Work out the finished part from the listing and answer in its coordinate system (mm). Face numbers are marked on the shaded views. A direction names the side the tool comes from. Give positions to 0.01 mm unless a question says otherwise; leave off trailing zeros. Order: outer loops, then holes, each group sorted by start corner. A loop starts at its lowest first (then second) coordinate and runs counter-clockwise, first axis right, second up. Notation, with made-up numbers: (-35, 24.5) -> (-15, 24.5) arc R21 cw to (-15, 38.5) -> close; hole circle Ø9 at (-28.75, 32.25). An arc over 180 degrees is marked (long way). Use a Markdown table: item, result. Add a question column.
```python
from build123d import *

# Parameters (mm, degrees)
CROQUIS3_W            = 395
CROQUIS3_H            = 35
REVOLUCI_N1_ANGLE     = 90
CROQUIS5_W            = 35
CROQUIS5_H            = 35
REVOLUCI_N3_ANGLE     = 90
CORTAR_EXTRUIR5_DEPTH = 360


with BuildPart() as part:
    # Croquis3 → Revolución1 (revolve)
    with BuildSketch(Plane(origin=(0, 0, 0), x_dir=(0, 0, -1), z_dir=(1, 0, 0))):
        with Locations((-727.916095406, 391.262754858)):
            Rectangle(CROQUIS3_W, CROQUIS3_H)
    revolve(axis=Axis((0, 408.762754858, 925.416095406), (0, -1, 0)), revolution_arc=REVOLUCI_N1_ANGLE)

    # Croquis5 → Revolución3 (revolve)
    with BuildSketch(Plane(origin=(0, 0, 0), x_dir=(0, 0, -1), z_dir=(1, 0, 0))):
        with Locations((-547.916095406, 426.262754858)):
            Rectangle(CROQUIS5_W, CROQUIS5_H)
    revolve(axis=Axis((0, 408.762754858, 925.416095406), (0, -1, 0)), revolution_arc=REVOLUCI_N3_ANGLE)

    # Croquis17 → Cortar-Extruir5 (cut)
    with BuildSketch(Plane.ZY):
        Polygon((925.416095406, 373.762754858), (900.416095406, 373.762754858), (925.416095406, 408.762754858), align=None)
    extrude(amount=-CORTAR_EXTRUIR5_DEPTH, mode=Mode.SUBTRACT)


solid = part.part
```
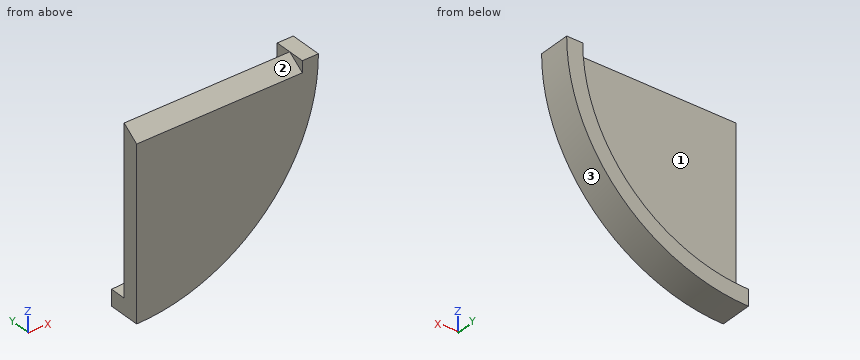
1) Which of the six approach directions +Z, -Z, +X, -X, +Y, -Y give full straight-line access (tool end or side, diameter ignored) to the marked faces 1, 2 and 3?
2) Straight lines are drawn through the part: line 1 (Y direction, x = 248, z = 844); line 2 (X direction, y = 387.5, z = 763); line 3 (X direction, y = 422.5, z = 635). For each, find the intervals that lie inside material, in ascending order.
3) The part is cut by section D-D, the plane y = 438. Determine the outline of the cut face in (x, z).
4) Flat-ended cylindrical pins translate along their axes: pin 1 (5 mm diameter, centred on x = 323, y = 390, fed in from +Z); pin 2 (4 mm diameter, centred on x = 268, y = 406, fed in from -Z); pin 3 (10 mm diameter, centred on x = 129.5, y = 415.5, fed in from +Z); pin 4 (1 mm diameter, centred on y = 401, z = 757, fed in from -X). Find the tip coordinate at first contact, or state that the pin passes through.
5) The part is cut by section C-C, the plane x = 312. Determine the outline of the cut face in (y, z).
6) The part is cut by section B-B, the plane z = 661. Determine the outline of the cut face in (x, y), then the cut area to 3 significant figures.
7) The part is cut by section A-A, the plane y = 386. Determine the outline of the cut face in (x, z).
A:
| question | item | result |
|---|---|---|
| 1 | face 1 | +Z, -X, +Y |
| 1 | face 2 | +Z, -X, -Y |
| 1 | face 3 | -Z, +X, +Y, -Y |
| 2 | line 1 | 373.76 to 408.76 |
| 2 | line 2 | 0 to 360.06 |
| 2 | line 3 | 212.74 to 267.74 |
| 3 | outline | (0, 530.42) arc R395 ccw to (395, 925.42) -> (360, 925.42) arc R360 cw to (0, 565.42) -> close |
| 4 | pin 1 | z = 913.8 |
| 4 | pin 2 | z = 633.41 |
| 4 | pin 3 | z = 591.49 |
| 4 | pin 4 | x = 0 |
| 5 | outline | (373.76, 683.17) -> (443.76, 683.17) -> (443.76, 745.82) -> (408.76, 745.82) -> (408.76, 925.42) -> (373.76, 900.42) -> close |
| 6 | outline | (0, 373.76) -> (293.44, 373.76) -> (293.44, 443.76) -> (244.3, 443.76) -> (244.3, 408.76) -> (0, 408.76) -> close |
| 6 | area | 12,000 mm^2 |
| 7 | outline | (0, 530.42) arc R395 ccw to (395, 925.42) -> (360, 925.42) -> (360, 909.16) -> (0, 909.16) -> close |
